Study the drawing (mm; zero at the part's minimum x, y, z) and answer. Coordinates: 2 decimals unless noted, no trailing zeros. Order: outer loops, then holes, each group sorted by start corner. A loop starts at its lowest first (then second) coordinate and runs counter-clockwise, first axis right, second up.
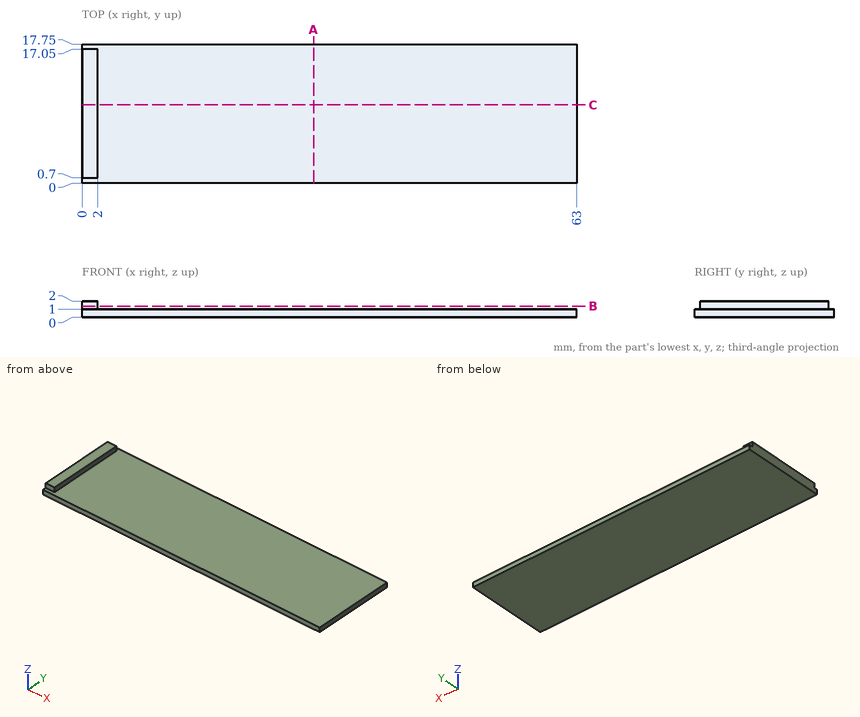
1) A cutting plane is placed at A-A, the plane x = 29.5. Determine the outline of the cut face in (y, z), and give its area (4 significant figures).
A:
outline: (0, 0) - (17.75, 0) - (17.75, 1) - (0, 1) - close
area: 17.75 mm2
2) A cutting plane is placed at C-C, the plane y = 10. Determine the outline of the cut face in (x, z), and give its area (3 significant figures).
A:
outline: (0, 0) - (63, 0) - (63, 1) - (2, 1) - (2, 2) - (0, 2) - close
area: 65.0 mm2
3) A cutting plane is placed at B-B, the plane z = 1.4. Determine the outline of the cut face in (x, y).
A:
outline: (0, 0.7) - (2, 0.7) - (2, 17.05) - (0, 17.05) - close
4) Straight lines are drawn through the part: line 1 (Z direction, x = 4.5, y = 6); line 2 (X direction, y = 12.5, z = 1.1). For each, find the intervals that lie inside material, in ascending order.
A:
line 1: z = 0 to 1
line 2: x = 0 to 2
5) Flat-ended cylindrical pins translate along their axes: pin 1 Ø0.5 at (x, z) = (1, 1.5) entering from +Y; pin 2 Ø5.5 at (x, y) = (36, 8) entering from +Z; pin 3 Ø0.5 at (x, z) = (1, 1.5) entering from -Y. Find the tip coordinate at first contact, or state that the pin passes through.
A:
pin 1: stops at y = 17.05
pin 2: stops at z = 1
pin 3: stops at y = 0.7
